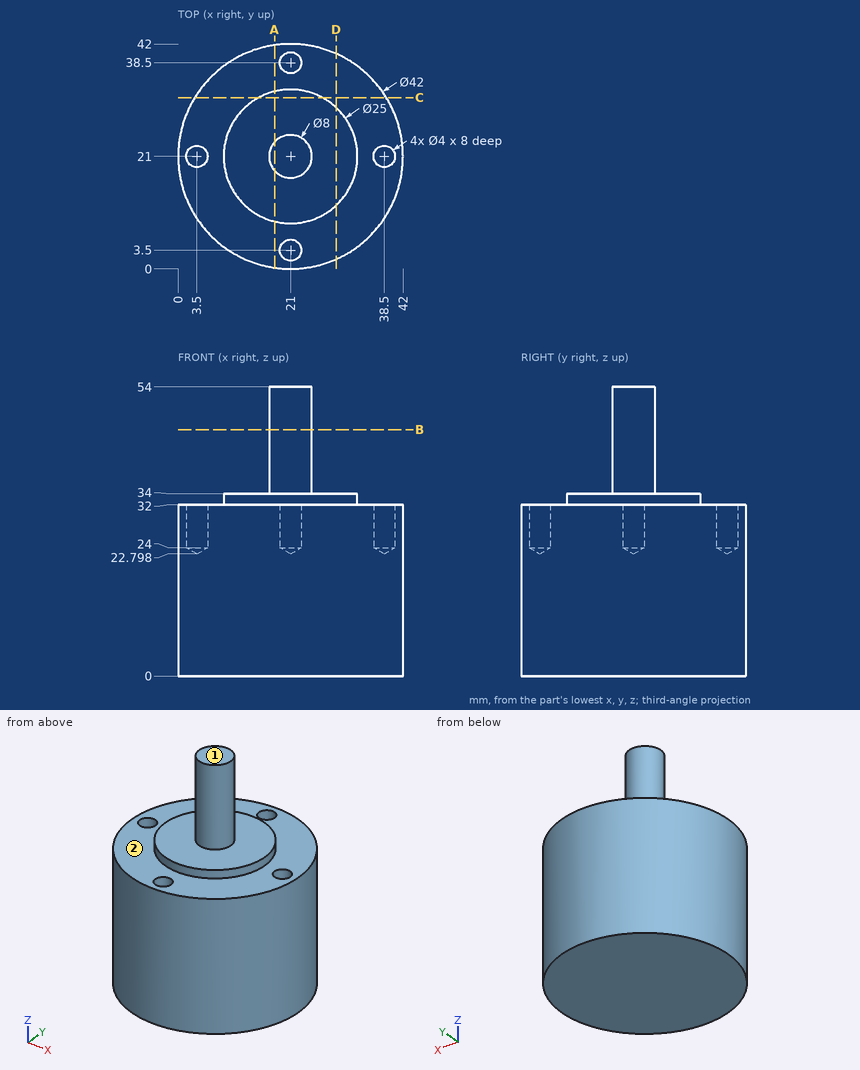
Geometry: see drawing. Coordinates: mm, zero at the bounding-box minimum. A direction names the side the tool comes from. Coordinates: 2 decimals unless noted, no trailing zeros. Loops run counter-clockwise (first coordinate to the right, second up) from the corner with the lowest first, then second, coordinate; pieces in that order, holes last. Notation, with made-up numbers: (-4, -24) -> (2, -24) arc R30 cw to (2, 10) -> close; hole circle Ø2 at (54.5, -29). An arc over 180 degrees is marked (long way). Write item = value, one per line. Start each with the question number.
Item 1: First-contact query: P1, Ø4, axis at x = 11.5, z = 20, coming from the +Y side (1 decimal); P2, Ø12, axis at y = 4.5, z = 37, coming from the -X side (1 decimal); P3, Ø1, axis at x = 9, y = 10, coming from the -Z side; P4, Ø4.5, axis at x = 21, y = 3.5, coming from the +Z side. Flat tips, straight axial feed; report the tip coordinate or a pass-through.
Item 2: Reachability of the marked faces 1 and 2 from +Z, -Z, +X, -X, +Y, -Y: full face, straight path, thin tool, end or side. Return the list, or none.
Item 3: Material intervals for line 1 (Y direction, x = 21, z = 30.5); line 2 (Z direction, x = 40, y = 25.5); line 3 (Z direction, x = 11.5, y = 20), sorted ascending.
Item 4: Cut plane B-B, the plane z = 46. Return loops of the section in (x, y), plus the area to 3 significant figures.
Item 5: Cut plane D-D, the plane x = 29.5. Return loops of the section in (y, z) (1 decimal).
Item 6: Cut plane A-A, the plane x = 18. Return loops of the section in (y, z) (1 decimal).
Item 7: Cut plane C-C, the plane y = 32. Return loops of the section in (x, z), plus the area to 3 significant figures.
Ans:
q1.P1 = 40.6
q1.P2 = 4.7
q1.P3 = 0
q1.P4 = 32
q2.face_1 = +Z, +X, -X, +Y, -Y
q2.face_2 = +Z
q3.line_1 = 0 to 1.5, 5.5 to 36.5, 40.5 to 42
q3.line_2 = 0 to 32
q3.line_3 = 0 to 34
q4.outline = circle Ø8 at (21, 21)
q4.area = 50.3 mm²
q5.outline = (1.8, 0) -> (40.2, 0) -> (40.2, 32) -> (30.2, 32) -> (30.2, 34) -> (11.8, 34) -> (11.8, 32) -> (1.8, 32) -> close
q6.outline = (0.2, 0) -> (41.8, 0) -> (41.8, 32) -> (33.1, 32) -> (33.1, 34) -> (23.6, 34) -> (23.6, 54) -> (18.4, 54) -> (18.4, 34) -> (8.9, 34) -> (8.9, 32) -> (0.2, 32) -> close
q7.outline = (3.11, 0) -> (38.89, 0) -> (38.89, 32) -> (26.94, 32) -> (26.94, 34) -> (15.06, 34) -> (15.06, 32) -> (3.11, 32) -> close
q7.area = 1,170 mm²
